Can you work these out from the drawing? Everything is in mm from the part's minimum corner. A direction names the side the tool comes from. Round coordinates to 2 decimals unless told otherwise and drop trailing zeros. Write each loop counter-clockwise with the first axis right and the second up, starting at its lowest first coordinate (ties: lowest second). Pieces come first, ordered by that corner, then holes. Notation, with made-up numbers: (4, 45.25) - (62, 45.25) arc R7 cw to (62, 49.25) - close; hole circle Ø5 at (0.25, -23). An arc over 180 degrees is marked (long way). Write each question's results on one line, items separated by ' | '. Start each with the question number.
(1) Imagine slicing it at D-D on z = 2. Write out the boundary of the cut face in (x, y), then the cut area to 3 significant figures.
(2) Imagine slicing it at B-B on y = 7.5. Write out the boundary of the cut face in (x, z).
(3) On a 3-axis mill with a long thin cutter (end or side, diameter ignored), from which of +Z, -Z, +X, -X, +Y, -Y can I reach the whole of each face in a straight line? I mean the marked faces 5, 6 and 7. Say none if no direction works.
(4) For P1, Ø1.2, axis at x = 1.5, y = 5, coming from the +Z side; P2, Ø5, axis at x = 8, y = 12, coming from the +Z side; P3, Ø8, axis at x = 22, y = 7.5, coming from the +Z side, each with a flat end and sliding along its axis, tell me the tip position at first contact or that it passes through.
(5) Thinking about a two-plate mould opening in Y: for the marked faces 1, 2, 3 and 4, which applies, +Y half, -Y half, draft (parallel to the pull), parting line (faces both ways), or undercut?
(6) Imagine slicing it at A-A on z = 20.5. Write out the boundary of the cut face in (x, y), then the cut area to 3 significant figures.
(7) Imagine slicing it at C-C on x = 8. Write out the boundary of the cut face in (y, z).
(8) Please list where these lines run through material, in increasing order: line 1 (Z direction, x = 28.75, y = 1); line 2 (X direction, y = 13.75, z = 8.25); line 3 (Y direction, x = 8, z = 2.8). Write a range as [from, to].
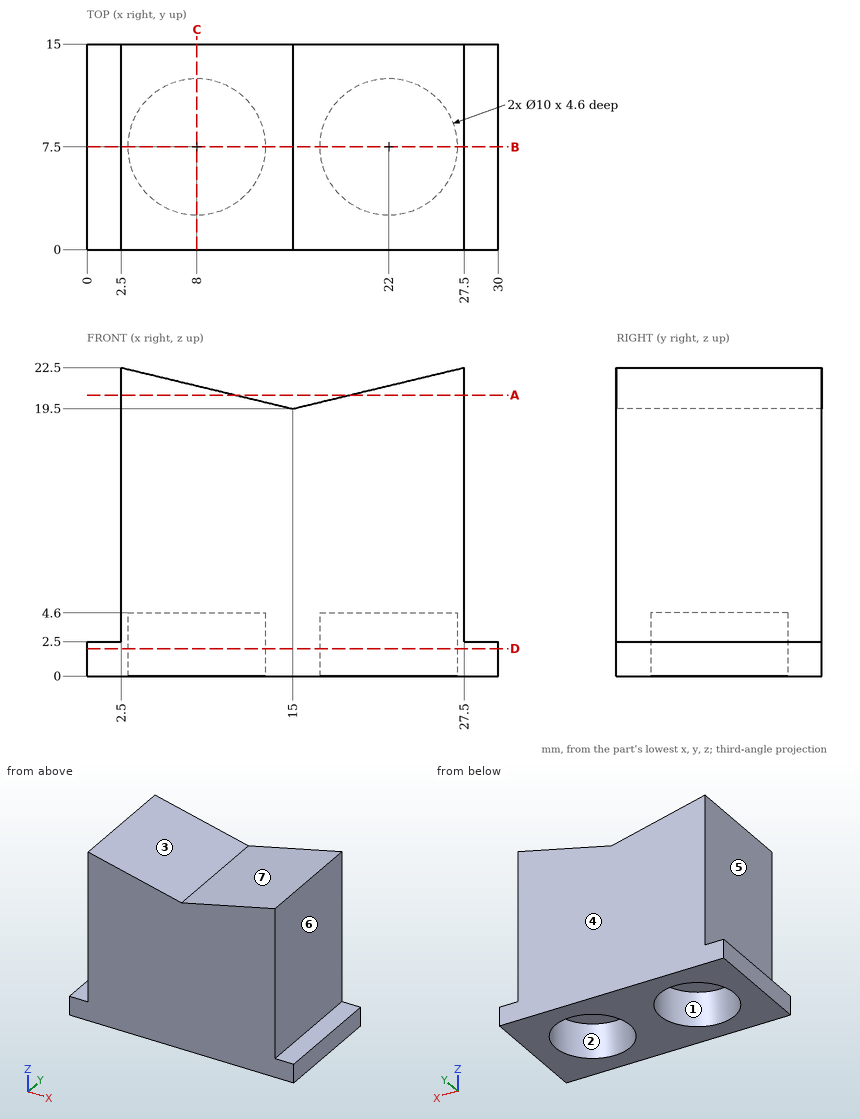
Response:
1) outline: (0, 0) - (30, 0) - (30, 15) - (0, 15) - close; hole circle Ø10 at (8, 7.5); hole circle Ø10 at (22, 7.5) | area: 293 mm²
2) outline: (0, 0) - (3, 0) - (3, 4.6) - (13, 4.6) - (13, 0) - (17, 0) - (17, 4.6) - (27, 4.6) - (27, 0) - (30, 0) - (30, 2.5) - (27.5, 2.5) - (27.5, 22.5) - (15, 19.5) - (2.5, 22.5) - (2.5, 2.5) - (0, 2.5) - close
3) face 5: +Z, -X, +Y, -Y | face 6: +Z, +X, +Y, -Y | face 7: +Z, +Y, -Y
4) P1: z = 2.5 | P2: z = 21.78 | P3: z = 22.14
5) face 1: undercut | face 2: undercut | face 3: draft | face 4: +Y half
6) outline: (2.5, 0) - (10.83, 0) - (10.83, 15) - (2.5, 15) - close; (19.17, 0) - (27.5, 0) - (27.5, 15) - (19.17, 15) - close | area: 250 mm²
7) outline: (0, 0) - (2.5, 0) - (2.5, 4.6) - (12.5, 4.6) - (12.5, 0) - (15, 0) - (15, 21.18) - (0, 21.18) - close
8) line 1: [0, 2.5] | line 2: [2.5, 27.5] | line 3: [0, 2.5], [12.5, 15]
